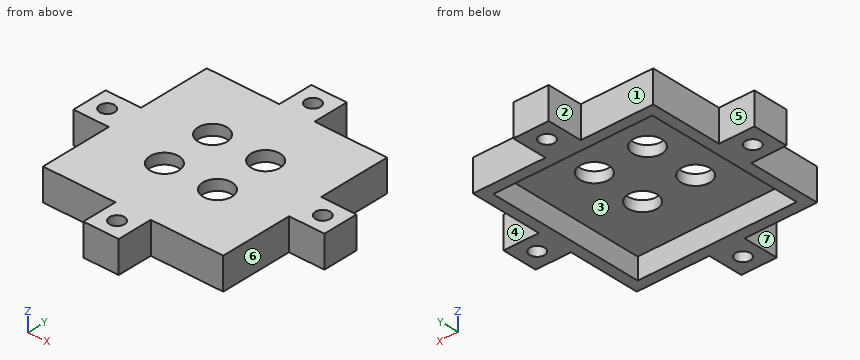
from build123d import *

# Parameters (mm, degrees)
F0_W     = 45
F0_H     = 45
F0_R     = 4.1
F1_DEPTH = 3
F2_W     = 51
F2_H     = 51
F2_W_2   = 45
F2_H_2   = 45
F3_DEPTH = 9
F4_W     = 10
F4_H     = 10
F4_R     = 2.1
F5_DEPTH = 9


with BuildPart() as f1:
    # F0 (on Top) → F1 (new body)
    with BuildSketch(Plane.XY):
        Rectangle(F0_W, F0_H)
        with Locations((-7.5, -7.5)):
            Circle(F0_R, mode=Mode.SUBTRACT)
        with Locations((7.5, -7.5)):
            Circle(F0_R, mode=Mode.SUBTRACT)
        with Locations((-7.5, 7.5)):
            Circle(F0_R, mode=Mode.SUBTRACT)
        with Locations((7.5, 7.5)):
            Circle(F0_R, mode=Mode.SUBTRACT)
    extrude(amount=F1_DEPTH)

    # F2 (on face) → F3 (join)
    with BuildSketch(Plane.XY.offset(3)):
        Rectangle(F2_W, F2_H)
        Rectangle(F2_W_2, F2_H_2, mode=Mode.SUBTRACT)
    extrude(amount=-F3_DEPTH)

    # F4 (on face) → F5 (join)
    with BuildSketch(Plane.XY.offset(3)):
        with Locations((0, 30.5)):
            Rectangle(F4_W, F4_H)
        with Locations((0, 30.5)):
            Circle(F4_R, mode=Mode.SUBTRACT)
        with Locations((-30.5, 0)):
            Rectangle(F4_W, F4_H)
        with Locations((-30.5, 0)):
            Circle(F4_R, mode=Mode.SUBTRACT)
        with Locations((0, -30.5)):
            Rectangle(F4_W, F4_H)
        with Locations((0, -30.5)):
            Circle(F4_R, mode=Mode.SUBTRACT)
        with Locations((30.5, 0)):
            Rectangle(F4_W, F4_H)
        with Locations((30.5, 0)):
            Circle(F4_R, mode=Mode.SUBTRACT)
    extrude(amount=-F5_DEPTH)


solid = f1.part
Build history of the part. All positions in model axes, mm. Face numbers are marked on the shaded views. A direction names the side the tool comes from. Give positions to 0.01 mm unless a question says otherwise; leave off trailing zeros. Order: outer loops, then holes, each group sorted by start corner. A loop starts at its lowest first (then second) coordinate and runs counter-clockwise, first axis right, second up. Notation, with made-up numbers: M 19,42.25 L 37,42.25 A19 cw 37,48.25 Z; hole C 64,65 d9. An arc over 180 degrees is marked long. Use one line per item in the form item = value.
1) Saw through at B-B (x = -30.5). Give the cut face in (y, z), plus the area to 3 significant figures.
Calculated:
outline = M -5,-6 L -2.1,-6 L -2.1,3 L -5,3 Z; M 2.1,-6 L 5,-6 L 5,3 L 2.1,3 Z
area = 52.2 mm2
2) Drop flat-ended pins along their axis: pin 1 (5 mm diameter, centred on y = 10, z = -4, fed in from +X); pin 2 (2 mm diameter, centred on x = 25, z = -0.5, fed in from +Y); pin 3 (2.5 mm diameter, centred on x = 17, z = -2.5, fed in from -Y); pin 4 (5 mm diameter, centred on x = 7.5, y = 7.5, fed in from +Z). Give the stop position or say it passes through.
Calculated:
pin_1 = 25.5
pin_2 = 25.5
pin_3 = -25.5
pin_4 = through
3) Tool access for the marked faces 4, 5, 6 and 7: list every direction of +Z, -Z, +X, -X, +Y, -Y with a clear straight run to the whole face (end or side of a thin tool).
Calculated:
face_4 = +Z, -Z, +X, +Y
face_5 = +Z, -Z, -X, +Y
face_6 = +Z, -Z, +X, -Y
face_7 = +Z, -Z, -X, -Y
4) Saw through at A-A (y = 0). Give the cut face in (x, z).
Calculated:
outline = M -35.5,-6 L -32.6,-6 L -32.6,3 L -35.5,3 Z; M -28.4,-6 L -22.5,-6 L -22.5,0 L 22.5,0 L 22.5,-6 L 28.4,-6 L 28.4,3 L -28.4,3 Z; M 32.6,-6 L 35.5,-6 L 35.5,3 L 32.6,3 Z
5) Two-plate mould, pull along Y, no slides. Class the marked faces 1, 2 and 3: released by +Y, released by -Y, zero draft, split by the parting line, or undercut.
Calculated:
face_1 = released by +Y
face_2 = zero draft
face_3 = undercut
6) Saw through at D-D (z = 2). State how many separate pieces and enclosed holes the cut face has, plus the area to 3 significant figures.
Calculated:
separate_pieces = 1
enclosed_holes = 8
area = 2,730 mm2
7) Probe probe 1 along Y at (x, z) = (-7.5, 0.7); probe 2 along Y at (x, z) = (0, 1); probe 3 along Y at (x, z) = (-30.5, 0.25). List the from-to ranges inside material, lowest first.
Calculated:
probe_1 = -25.5 to -11.6, -3.4 to 3.4, 11.6 to 25.5
probe_2 = -35.5 to -32.6, -28.4 to 28.4, 32.6 to 35.5
probe_3 = -5 to -2.1, 2.1 to 5
8) Saw through at C-C (z = -2.25). Give the cut face in (x, y), plus the area to 3 significant figures.
Calculated:
outline = M -35.5,-5 L -25.5,-5 L -25.5,-25.5 L -5,-25.5 L -5,-35.5 L 5,-35.5 L 5,-25.5 L 25.5,-25.5 L 25.5,-5 L 35.5,-5 L 35.5,5 L 25.5,5 L 25.5,25.5 L 5,25.5 L 5,35.5 L -5,35.5 L -5,25.5 L -25.5,25.5 L -25.5,5 L -35.5,5 Z; hole C -30.5,0 d4.2; hole M -22.5,-22.5 L 22.5,-22.5 L 22.5,22.5 L -22.5,22.5 Z; hole C 0,-30.5 d4.2; hole C 0,30.5 d4.2; hole C 30.5,0 d4.2
area = 921 mm2
